Answer from the drawing. Dimensions are ordinates in mm from the lowest x, y and z of the part. A direction names the side the tool comes from. Coordinates: 2 decimals unless noted, no trailing zeros. Order: outer loops, then holes, each group sorted by start corner. A loop starts at its lowest first (then second) coordinate and runs counter-clockwise, first axis right, second up. Notation, with made-up numbers: (20, -38.5) -> (61, -38.5) arc R12 ccw to (61, -23.5) -> close; hole circle Ø7 at (16, 1). An arc over 180 degrees is marked (long way). Answer in a Markdown table with one row per item.
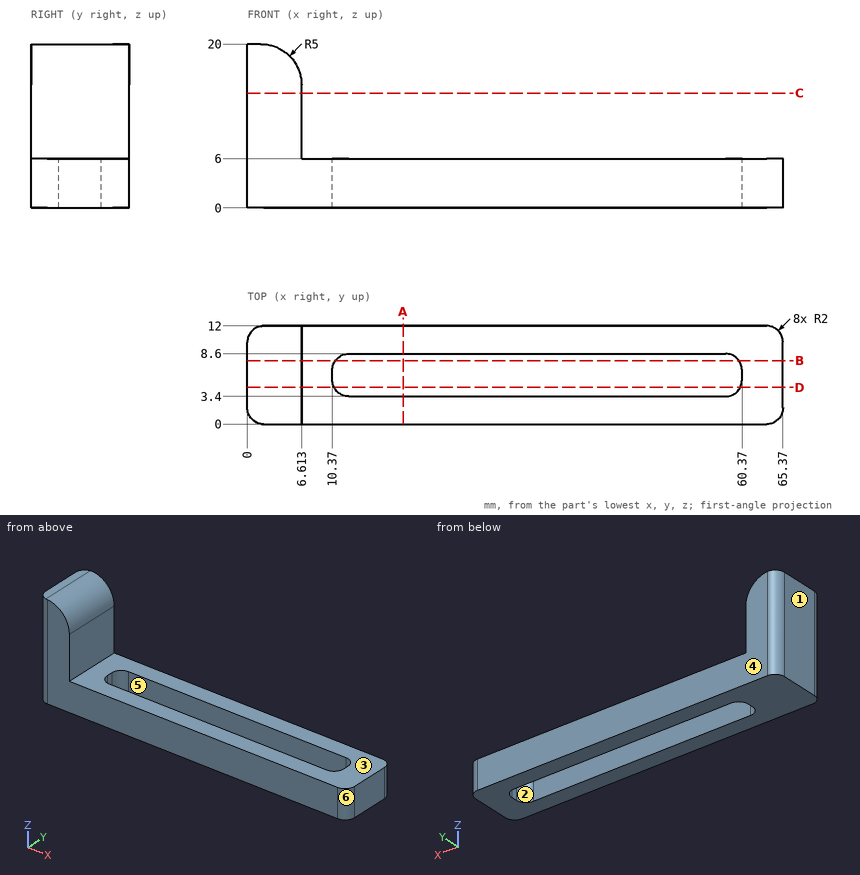
Q1. The part is cut by section B-B (y = 7.75). Write down the section's boundary in (x, z) (1 decimal).
Outcome:
| item | result |
|---|---|
| outline | (0, 0) -> (10.7, 0) -> (10.7, 6) -> (6.6, 6) -> (6.6, 15) arc R5 ccw to (1.6, 20) -> (0, 20) -> close; (60, 0) -> (65.4, 0) -> (65.4, 6) -> (60, 6) -> close |
Q2. Given pin 1 (4 mm diameter, centred on y = 2.5, z = 15.5, fed in from +X); pin 2 (5 mm diameter, centred on x = 42.5, y = 2, fed in from +Z), each flat-ended and moving along its own axis, determine where each tip first touches the part or whether it passes through.
Outcome:
| item | result |
|---|---|
| pin 1 | x = 6.61 |
| pin 2 | z = 6 |
Q3. The part is cut by section A-A (x = 19). Write down the section's boundary in (y, z), then the cut area to 3 significant figures.
Outcome:
| item | result |
|---|---|
| outline | (0, 0) -> (3.4, 0) -> (3.4, 6) -> (0, 6) -> close; (8.6, 0) -> (12, 0) -> (12, 6) -> (8.6, 6) -> close |
| area | 40.8 mm² |
Q4. Consider line 1 (Y direction, x = 15, z = 1.75); line 2 (X direction, y = 7.25, z = 1); line 3 (Z direction, x = 24, y = 9.75). Determine where each line is inside the solid, lowest interval first.
Outcome:
| item | result |
|---|---|
| line 1 | 0 to 3.4, 8.6 to 12 |
| line 2 | 0 to 10.48, 60.26 to 65.37 |
| line 3 | 0 to 6 |
Q5. The part is cut by section D-D (y = 4.5). Write down the section's boundary in (x, z) (1 decimal).
Outcome:
| item | result |
|---|---|
| outline | (0, 0) -> (10.6, 0) -> (10.6, 6) -> (6.6, 6) -> (6.6, 15) arc R5 ccw to (1.6, 20) -> (0, 20) -> close; (60.2, 0) -> (65.4, 0) -> (65.4, 6) -> (60.2, 6) -> close |
Q6. For a pull along X with two mould halves and no side action, classify the marked faces 4, 5 and 6 as pulls with the +X half, pulls with the -X half, needs draft (parallel to the pull), parting line crosses it, or undercut.
Outcome:
| item | result |
|---|---|
| face 4 | needs draft |
| face 5 | undercut |
| face 6 | pulls with the +X half |
Q7. The part is cut by section C-C (z = 14). Write down the section's boundary in (x, y).
Outcome:
| item | result |
|---|---|
| outline | (0, 2) arc R2 ccw to (2, 0) -> (6.61, 0) -> (6.61, 12) -> (2, 12) arc R2 ccw to (0, 10) -> close |
Q8. For the marked faces 1, 2 and 3, determine the directions among +Z, -Z, +X, -X, +Y, -Y from which every point of the face is accessible in a straight line to the end or side of a thin tool.
Outcome:
| item | result |
|---|---|
| face 1 | +Z, -Z, -X, +Y, -Y |
| face 2 | +Z, -Z |
| face 3 | +Z, +X, +Y, -Y |
